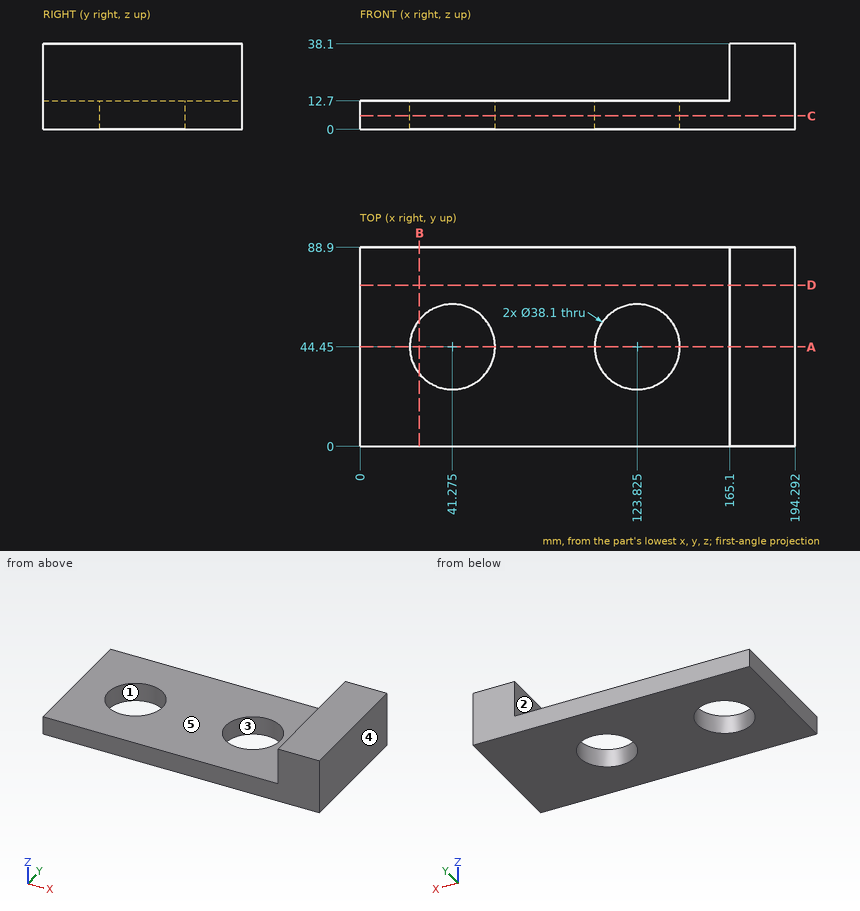
Here's the drawing with two shaded views (mm, measured from the low corner). I have some questions. A direction names the side the tool comes from. Give positions to 0.01 mm unless a question says otherwise; leave off trailing zeros. Write each loop counter-clockwise with the first axis right and the second up, starting at its lowest first coordinate (ties: lowest second). Pieces come first, ordered by that corner, then holes. Notation, with made-up numbers: (39, -40) -> (73, -40) arc R25 ccw to (73, -25) -> close; hole circle Ø8 at (-26.75, -24). An arc over 180 degrees is marked (long way). Answer as a JSON object with one key per item and string values. Group by question number.
Item 1: Suppose I cut it at D-D (y = 72). Please give me the cut outline in (x, z).
Item 2: Suppose I cut it at A-A (y = 44.45). Please give me the cut outline in (x, z) (1 decimal).
Item 3: Suppose I cut it at C-C (z = 6). State how many separate pieces and enclosed holes the cut face has, plus the area to 3 significant figures.
Item 4: I'm going to push a flat-ended pin straight in: P1, Ø8, axis at y = 31.5, z = 25.5, coming from the -X side. Where does the tip first touch, or does it pass through?
Item 5: For the marked faces 1 and 2, which set-ups out of +Z, -Z, +X, -X, +Y, -Y let a thin tool reach every point of the face, with its end or its side?
Item 6: We'd pull the mould along X, two halves only. Please class the marked faces 3, 4 and 5: +X half, -X half, draft (parallel to the pull), parting line (faces both ways), or undercut.
Item 7: Suppose I cut it at B-B (x = 26.5). Please give me the cut outline in (y, z) (1 decimal).
Item 8: Please list where these lines run through material, in increasing order: line 1 (X direction, y = 12.5, z = 32.5); line 2 (Z direction, x = 103, y = 39); line 3 (Y direction, x = 24, z = 2.5) (1 decimal). Write a range as [from, to].
Findings:
{
 "1": {"outline": "(0, 0) -> (194.29, 0) -> (194.29, 38.1) -> (165.1, 38.1) -> (165.1, 12.7) -> (0, 12.7) -> close"},
 "2": {"outline": "(0, 0) -> (22.2, 0) -> (22.2, 12.7) -> (0, 12.7) -> close; (60.3, 0) -> (104.8, 0) -> (104.8, 12.7) -> (60.3, 12.7) -> close; (142.9, 0) -> (194.3, 0) -> (194.3, 38.1) -> (165.1, 38.1) -> (165.1, 12.7) -> (142.9, 12.7) -> close"},
 "3": {"separate pieces": "1", "enclosed holes": "2", "area": "15,000 mm²"},
 "4": {"P1": "stops at x = 165.1"},
 "5": {"face 1": "+Z, -Z", "face 2": "+Z, -X, +Y, -Y"},
 "6": {"face 3": "undercut", "face 4": "+X half", "face 5": "draft"},
 "7": {"outline": "(0, 0) -> (32.4, 0) -> (32.4, 12.7) -> (0, 12.7) -> close; (56.5, 0) -> (88.9, 0) -> (88.9, 12.7) -> (56.5, 12.7) -> close"},
 "8": {"line 1": "x = [165.1, 194.29]", "line 2": "z = [0, 12.7]", "line 3": "y = [0, 36.4], [52.5, 88.9]"}
}
